Geometry: see drawing. Coordinates: mm, zero at the bounding-box minimum. Give positions to 0.01 mm unless a question says otherwise; leave off trailing zeros. Write each loop counter-clockwise with the first axis right and the second up, starting at its lowest first coordinate (ties: lowest second). Pieces come first, ordered by that corner, then holes. Notation, with made-up numbers: M 12.25,2 L 52.25,2 A16 ccw 52.25,6 Z; hole C -14.5,78.5 d1. An arc over 180 degrees is marked long. Answer as a JSON object with one key per item and string values. Group by question number.
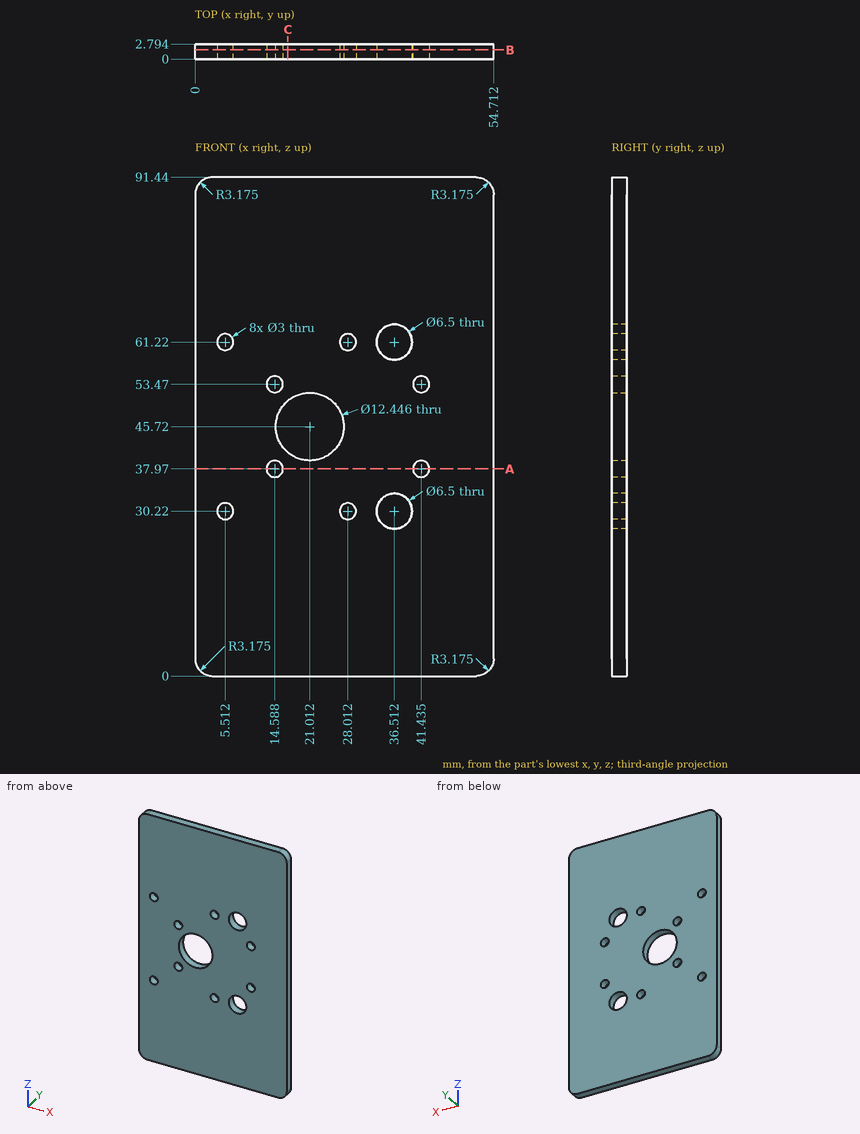
(1) Contact query for a flat-ended pin moving along its axis: pin 1 Ø2.5 at (x, z) = (28.01, 30.22) entering from +Y. Output: stop coordinate, or through.
(2) Section A-A, the plane z = 37.97. Return loops of the section in (x, y) (1 decimal).
(3) Section C-C, the plane x = 17. Return loops of the section in (y, z).
(4) Section B-B, the plane y = 1.7. State how many separate pieces and enclosed holes the cut face has, plus the area to 3 significant figures.
(5) Ray query, L1, parallel to Z at x = 28, y = 1.95; L2, parallel to X at y = 1.35, z = 37.97 (1 decimal); L3, parallel to X at y = 0.2, z = 29 (1 decimal). Return the intervals inside material, ascending. Write a range as [from, to].
Reported:
{
 "1": {"pin 1": "passes through"},
 "2": {"outline": "M 0,0 L 13.1,0 L 13.1,2.8 L 0,2.8 Z; M 16.1,0 L 39.9,0 L 39.9,2.8 L 16.1,2.8 Z; M 42.9,0 L 54.7,0 L 54.7,2.8 L 42.9,2.8 Z"},
 "3": {"outline": "M 0,0 L 2.79,0 L 2.79,40.96 L 0,40.96 Z; M 0,50.48 L 2.79,50.48 L 2.79,91.44 L 0,91.44 Z"},
 "4": {"separate pieces": "1", "enclosed holes": "11", "area": "4,750 mm2"},
 "5": {"L1": "z = [0, 28.72], [31.72, 59.72], [62.72, 91.44]", "L2": "x = [0, 13.1], [16.1, 39.9], [42.9, 54.7]", "L3": "x = [0, 4.6], [6.4, 27.1], [28.9, 33.5], [39.5, 54.7]"}
}
